```python
from build123d import *

# Parameters (mm, degrees)
SKETCH2_W           = 100
SKETCH2_H           = 40
BOSS_EXTRUDE1_DEPTH = 10
SKETCH3_R           = 7.5
CUT_EXTRUDE1_DEPTH  = 55.772255751
SKETCH4_R           = 16
CUT_EXTRUDE2_DEPTH  = 55.772255751
SKETCH5_R           = 2.5
BOSS_EXTRUDE2_DEPTH = 10


with BuildPart() as part:
    # Sketch2 → Boss-Extrude1 (new body)
    with BuildSketch(Plane.XY):
        Rectangle(SKETCH2_W, SKETCH2_H)
    extrude(amount=BOSS_EXTRUDE1_DEPTH)

    # Sketch3 → Cut-Extrude1 (cut, through all)
    with BuildSketch(Plane.XY.offset(10)):
        Circle(SKETCH3_R)
    extrude(amount=-CUT_EXTRUDE1_DEPTH, mode=Mode.SUBTRACT)

    # Sketch4 → Cut-Extrude2 (cut, through all)
    with BuildSketch(Plane.XY.offset(10)):
        Circle(SKETCH4_R)
    extrude(amount=-CUT_EXTRUDE2_DEPTH, mode=Mode.SUBTRACT)

    # Sketch5 → Boss-Extrude2 (add)
    with BuildSketch(Plane.ZY.offset(50)):
        Polygon((0, 20), (10, 20), (10, 15), (45, -20), (45, -32.5), (10, -32.5), (0, -32.5), align=None)
        with Locations((5, -27.5)):
            Circle(SKETCH5_R, mode=Mode.SUBTRACT)
        with Locations((40, -27.5)):
            Circle(SKETCH5_R, mode=Mode.SUBTRACT)
    boss_extrude2 = extrude(amount=BOSS_EXTRUDE2_DEPTH)

    # Mirror1: Boss-Extrude2 across plane
    add(boss_extrude2.mirror(Plane(origin=(0, 0, 0), x_dir=(0, 0, 1), z_dir=(1, 0, 0))))


solid = part.part
```
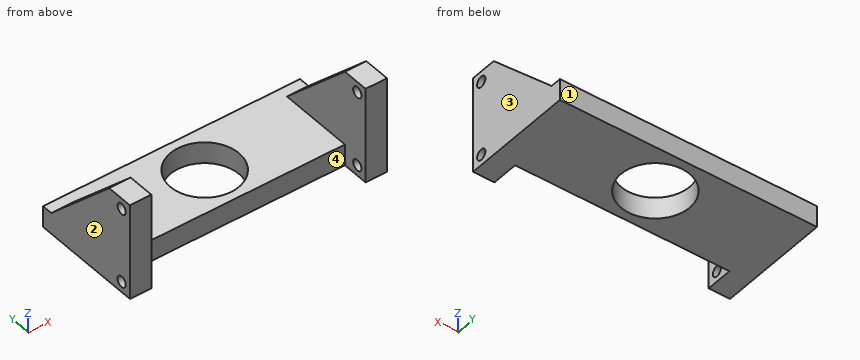
Verification items for the finished model (mm, model axes). Face numbers are marked on the shaded views. Give positions to 0.01 mm unless a question says otherwise; leave off trailing zeros. Loops run counter-clockwise (first coordinate to the right, second up) from the corner with the lowest first, then second, coordinate; pieces in that order, holes last. Notation, with made-up numbers: M -6.75,30.25 L 9.25,30.25 A38 ccw 9.25,68.25 Z; hole C -11.75,39.25 d6. An arc over 180 degrees is marked long. One line per question, with ' | ' between items.
Item 1: Draft check along X on the marked faces 1, 2, 3 and 4. Enter one of: +X half, -X half, draft (parallel to the pull), parting line (faces both ways), or undercut.
Completed:
face 1: draft | face 2: -X half | face 3: +X half | face 4: undercut
Item 2: Section check C-C, the plane y = -27.5. Record the cut outline in (x, z).
Completed:
outline: M -60,0 L -50,0 L -50,2.5 L -60,2.5 Z; M -60,7.5 L -50,7.5 L -50,37.5 L -60,37.5 Z; M -60,42.5 L -50,42.5 L -50,45 L -60,45 Z; M 50,0 L 60,0 L 60,2.5 L 50,2.5 Z; M 50,7.5 L 60,7.5 L 60,37.5 L 50,37.5 Z; M 50,42.5 L 60,42.5 L 60,45 L 50,45 Z
Item 3: Thickness scan on line 1 (X direction, y = 12, z = 10.5); line 2 (Y direction, x = 0, z = 4); line 3 (Z direction, x = -56, y = -27). Record the ranges inside material, lowest first. Write a range as [from, to].
Completed:
line 1: x = [-60, -50], [50, 60] | line 2: y = [-20, -16], [16, 20] | line 3: z = [0, 2.55], [7.45, 37.55], [42.45, 45]
Item 4: Section check D-D, the plane x = 0. Record the cut outline in (y, z), plus the area to 3 significant figures.
Completed:
outline: M -20,0 L -16,0 L -16,10 L -20,10 Z; M 16,0 L 20,0 L 20,10 L 16,10 Z | area: 80.0 mm^2
Item 5: Section check A-A, the plane y = 0. Record the cut outline in (x, z).
Completed:
outline: M -60,0 L -16,0 L -16,10 L -50,10 L -50,25 L -60,25 Z; M 16,0 L 60,0 L 60,25 L 50,25 L 50,10 L 16,10 Z
Item 6: Section check B-B, the plane z = 23. Record the cut outline in (x, y).
Completed:
outline: M -60,-32.5 L -50,-32.5 L -50,2 L -60,2 Z; M 50,-32.5 L 60,-32.5 L 60,2 L 50,2 Z
Item 7: Depth check by flat-ended pin: P1, Ø6, axis at x = 14, y = 11, coming from the +Z side; P2, Ø5, axis at x = -10.5, z = 3, coming from the -Y side; P3, Ø6, axis at y = -27.5, z = 40, coming from the +X side. Enter the tip coordinate at first touch or a pass-through.
Completed:
P1: stops at z = 10 | P2: stops at y = -20 | P3: stops at x = 60
